Input: part model. Units: mm. Frame: model coordinates. A direction names the side the tool comes from. Coordinates: 2 decimals unless noted, no trailing zeros. Write each loop counter-clockwise with the first axis right and the second up, starting at its lowest first coordinate (ties: lowest second). Pieces come first, ordered by that corner, then holes. Notation, with made-up numbers: (89, -38.5) - (99, -38.5) arc R18 cw to (99, -24.5) - close; hole circle Ø4 at (-10, 10.25). An arc over 180 degrees is marked (long way). Use a Markdown table: item, result. Add a question column.
Q1. Set-up query: faces 1 (the face through (35.475, 37.535, -37.578)), 2 (the face through (0, 21, -21)). Return all of +Z, -Z, +X, -X, +Y, -Y with unobstructed straight access to the full face (end or side cutting, diameter ignored); none if empty.
Q2. Mould query, pull axis Z, two halves, no side actions, for faces 3 (the face through (37, 35, -6)), 4 (the face through (21, 21, 0)), 5 (the face through (2, 21, -40.3)). Classes: released by +Z, released by -Z, zero draft, split by the parting line, or undercut.
Q3. Section query B-B (x = 21.15). Return the cut outline in (y, z), then the cut area to 3 significant figures.
Q4. Section query D-D (x = 30.5). Return the cut outline in (y, z), then the cut area to 3 significant figures.
Q5. Material intervals for probe 1 along Y at (x, z) = (18.5, -6.5); probe 2 along Y at (x, z) = (19, -27); probe 3 along X at (y, z) = (40.5, -19.5), sorted ascending. Write a range as from..to.
Q6. Section query A-A (y = 28). Return the cut outline in (x, z), then the cut area to 3 significant figures.
Q7. Pin query (flat end, axial travel): P1, Ø1.5, axis at x = 37, z = -36.5, coming from the +Y side; P2, Ø3, axis at x = 21.5, y = 53.5, coming from the -Z side; P3, Ø3.5, axis at x = 37, z = -5.5, coming from the +Y side. Return the tip coordinate at first contact, or that it passes through.
Q8. Section query C-C (z = -21.15). Return the cut outline in (x, y).
from build123d import *

# Parameters (mm, degrees)
BOSS_EXTRUDE1_DEPTH = 40
SKETCH2_R           = 1.5
CUT_EXTRUDE1_DEPTH  = 5
CHAMFER1_SIZE       = 0.35
D_SHAFT_DEPTH       = 22
CHAMFER2_SIZE       = 2.54


with BuildPart() as part:
    # Sketch1 → Boss-Extrude1 (new body)
    with BuildSketch(Plane(origin=(0, 0, 0), x_dir=(1, 0, 0), z_dir=(0, 1, 0))):
        Polygon((4, 42.3), (0, 38.3), (0, 4), (4, 0), (38.3, 0), (42.3, 4), (42.3, 38.3), (38.3, 42.3), align=None)
    extrude(amount=BOSS_EXTRUDE1_DEPTH)

    # Sketch2 → Cut-Extrude1 (cut)
    with BuildSketch(Plane.XZ.offset(-40)):
        with Locations((5.635, -5.635)):
            Circle(SKETCH2_R)
        with Locations((36.665, -5.635)):
            Circle(SKETCH2_R)
        with Locations((36.665, -36.665)):
            Circle(SKETCH2_R)
        with Locations((5.635, -36.665)):
            Circle(SKETCH2_R)
    extrude(amount=CUT_EXTRUDE1_DEPTH, mode=Mode.SUBTRACT)

    # Sketch6 → Revolve1 (revolve)
    with BuildSketch(Plane.XY.offset(-21.15)):
        Polygon((21.15, 40), (32.15, 40), (32.15, 42), (23.65, 42), (23.65, 64), (21.15, 64), align=None)
    revolve(axis=Axis((21.15, 64, -21.15), (0, -1, 0)))

    # Chamfer1
    chamfer1_edges = [part.edges().sort_by_distance(p)[0] for p in [
        (18.65, 64, -21.15),
    ]]
    chamfer(chamfer1_edges, length=CHAMFER1_SIZE)

    # Sketch7 → D shaft (cut)
    with BuildSketch(Plane(origin=(0, 64, 0), x_dir=(1, 0, 0), z_dir=(0, 1, 0))):
        with BuildLine():
            Line((22.621309131, 23.1712), (19.678690869, 23.1712))
            ThreePointArc((19.678690869, 23.1712), (21.15, 23.65), (22.621309131, 23.1712))
        make_face()
    extrude(amount=-D_SHAFT_DEPTH, mode=Mode.SUBTRACT)

    # Chamfer2
    chamfer2_edges = [part.edges().sort_by_distance(p)[0] for p in [
        (2, 0, -40.3),
        (21.15, 0, -42.3),
        (40.3, 0, -40.3),
        (42.3, 0, -21.15),
        (40.3, 0, -2),
        (21.15, 0, 0),
        (2, 0, -2),
        (0, 0, -21.15),
    ]]
    chamfer(chamfer2_edges, length=CHAMFER2_SIZE)


solid = part.part
Values follow:
| question | item | result |
|---|---|---|
| 1 | face 1 | +Y |
| 1 | face 2 | +Z, -Z, -X, +Y, -Y |
| 2 | face 3 | undercut |
| 2 | face 4 | released by +Z |
| 2 | face 5 | released by -Z |
| 3 | outline | (0, -39.76) - (2.54, -42.3) - (40, -42.3) - (40, -32.15) - (42, -32.15) - (42, -23.17) - (64, -23.17) - (64, -19) - (63.65, -18.65) - (42, -18.65) - (42, -10.15) - (40, -10.15) - (40, 0) - (2.54, 0) - (0, -2.54) - close |
| 3 | area | 1,830 mm2 |
| 4 | outline | (0, -39.76) - (2.54, -42.3) - (40, -42.3) - (40, -26.94) - (42, -26.94) - (42, -15.36) - (40, -15.36) - (40, 0) - (2.54, 0) - (0, -2.54) - close |
| 4 | area | 1,710 mm2 |
| 5 | probe 1 | 0..40 |
| 5 | probe 2 | 0..42 |
| 5 | probe 3 | 10.27..32.03 |
| 6 | outline | (0, -38.3) - (4, -42.3) - (38.3, -42.3) - (42.3, -38.3) - (42.3, -4) - (38.3, 0) - (4, 0) - (0, -4) - close |
| 6 | area | 1,760 mm2 |
| 7 | P1 | y = 35 |
| 7 | P2 | z = -23.17 |
| 7 | P3 | y = 40 |
| 8 | outline | (0, 2.54) - (2.54, 0) - (39.76, 0) - (42.3, 2.54) - (42.3, 40) - (32.15, 40) - (32.15, 42) - (23.65, 42) - (23.65, 63.65) - (23.3, 64) - (19, 64) - (18.65, 63.65) - (18.65, 42) - (10.15, 42) - (10.15, 40) - (0, 40) - close |
